The model under review builds one solid part; all positions refer to its coordinate system, in mm. A direction names the side the tool comes from. Round coordinates to 2 decimals unless told otherwise and drop trailing zeros. Order: outer loops, then holes, each group sorted by start corner. A loop starts at its lowest first (then second) coordinate and runs counter-clockwise, first axis right, second up. Notation, with made-up numbers: (65, -3.5) -> (69, -3.5) arc R36 ccw to (69, 35.5) -> close; hole circle Ø1 at (66.5, 68.25). An arc over 180 degrees is marked (long way). Use a Markdown table: item, result. Add a question column.
```python
from build123d import *

# Parameters (mm, degrees)
SKETCH1_R             = 24
SKETCH1_R_2           = 20
BOSS_EXTRUDE1_DEPTH   = 10
BOSS_EXTRUDE1_2_DEPTH = 10
BOSS_EXTRUDE1_3_DEPTH = 10
BOSS_EXTRUDE1_4_DEPTH = 10
BOSS_EXTRUDE2_DEPTH   = 3
SKETCH3_W             = 121.220550743
SKETCH3_H             = 101.763820318
CUT_EXTRUDE1_DEPTH    = 10
SKETCH4_R             = 4.5
BOSS_EXTRUDE4_DEPTH   = 5
FILLET1_R             = 10


with BuildPart() as part:
    # Sketch1 → Boss-Extrude1 (new body)
    with BuildSketch(Plane(origin=(0, 0, 0), x_dir=(1, 0, 0), z_dir=(0, 1, 0))):
        with Locations(Location((-28, -48.497422612, 0), (0, 0, 270))):
            Circle(SKETCH1_R)
        with Locations(Location((-28, -48.497422612, 0), (0, 0, 270))):
            Circle(SKETCH1_R_2, mode=Mode.SUBTRACT)
    extrude(amount=BOSS_EXTRUDE1_DEPTH)



with BuildPart() as body_2:
    # Sketch1 → Boss-Extrude1 2 (new body)
    with BuildSketch(Plane(origin=(0, 0, 0), x_dir=(1, 0, 0), z_dir=(0, 1, 0))):
        with Locations(Location((0, 0, 0), (0, 0, 270))):
            Circle(SKETCH1_R)
        with Locations(Location((0, 0, 0), (0, 0, 270))):
            Circle(SKETCH1_R_2, mode=Mode.SUBTRACT)
    extrude(amount=BOSS_EXTRUDE1_2_DEPTH)


with BuildPart() as body_3:
    # Sketch1 → Boss-Extrude1 3 (new body)
    with BuildSketch(Plane(origin=(0, 0, 0), x_dir=(1, 0, 0), z_dir=(0, 1, 0))):
        with Locations(Location((28, -48.497422612, 0), (0, 0, 270))):
            Circle(SKETCH1_R)
        with Locations(Location((28, -48.497422612, 0), (0, 0, 270))):
            Circle(SKETCH1_R_2, mode=Mode.SUBTRACT)
    extrude(amount=BOSS_EXTRUDE1_3_DEPTH)


with BuildPart() as body_4:
    # Sketch1 → Boss-Extrude1 4 (new body)
    with BuildSketch(Plane(origin=(0, 0, 0), x_dir=(1, 0, 0), z_dir=(0, 1, 0))):
        with BuildLine():
            ThreePointArc((4.672620947, -29.633876113), (2.019237886, -33.497422612), (0, -37.727092998))
            ThreePointArc((0, -37.727092998), (-2.019237886, -33.497422612), (-4.672620947, -29.633876113))
            ThreePointArc((-4.672620947, -29.633876113), (0, -30), (4.672620947, -29.633876113))
        make_face()
    extrude(amount=BOSS_EXTRUDE1_4_DEPTH)


with BuildPart() as part_1:
    add(part.part)

    add(body_2.part)  # Boss-Extrude2 merges body 2

    add(body_3.part)  # Boss-Extrude2 merges body 3

    add(body_4.part)  # Boss-Extrude2 merges body 4
    # Sketch2 → Boss-Extrude2 (add)
    with BuildSketch(Plane(origin=(0, 10, 0), x_dir=(1, 0, 0), z_dir=(0, 1, 0))):
        with BuildLine():
            Line((-20, -32.516950024), (-20, -56.505922275))
            Line((-20, -56.505922275), (20, -56.505922275))
            Line((20, -56.505922275), (20, -32.516950024))
            ThreePointArc((20, -32.516950024), (0, -12.516950024), (-20, -32.516950024))
        make_face()
    extrude(amount=BOSS_EXTRUDE2_DEPTH)

    # Sketch3 → Cut-Extrude1 (cut)
    with BuildSketch(Plane.XZ):
        with Locations((1.216045651, 23.416680071)):
            Rectangle(SKETCH3_W, SKETCH3_H)
        Polygon((0, 0), (28, 48.497422612), (-28, 48.497422612), align=None, mode=Mode.SUBTRACT)
    extrude(amount=-CUT_EXTRUDE1_DEPTH, mode=Mode.SUBTRACT)

    # Sketch4 → Boss-Extrude4 (add)
    with BuildSketch(Plane(origin=(0, 13, 0), x_dir=(1, 0, 0), z_dir=(0, 1, 0))):
        with Locations(Location((0, -32.516950024, 0), (0, 0, 270))):
            Circle(SKETCH4_R)
        with BuildLine():
            Line((-10, -18.516950024), (10, -18.516950024))
            ThreePointArc((10, -18.516950024), (11.4, -19.916950024), (10, -21.316950024))
            Line((10, -21.316950024), (-10, -21.316950024))
            ThreePointArc((-10, -21.316950024), (-11.4, -19.916950024), (-10, -18.516950024))
        make_face()
        with BuildLine():
            Line((-15, -49.516950024), (15, -49.516950024))
            ThreePointArc((15, -49.516950024), (16.4, -50.916950024), (15, -52.316950024))
            Line((15, -52.316950024), (-15, -52.316950024))
            ThreePointArc((-15, -52.316950024), (-16.4, -50.916950024), (-15, -49.516950024))
        make_face()
    extrude(amount=BOSS_EXTRUDE4_DEPTH)

    # Fillet1
    fillet1_edges = [part_1.edges().sort_by_distance(p)[0] for p in [
        (-20, 11.5, 56.505922275),
        (20, 11.5, 56.505922275),
    ]]
    fillet(fillet1_edges, radius=FILLET1_R)


solid = part_1.part
```
Q1. Mouldability with a two-part tool opening along X and no side actions: class faces 5 (the flat face through (0, 15, 49.517)), 6 (the flat face through (-11.014, 4.93, 19.077)), 7 (the cylindrical face through (7.3, 4.93, 36.35)) as pulls with the +X half, pulls with the -X half, needs draft (parallel to the pull), parting line crosses it, or undercut.
Q2. Add section B-B (y = 8.25). Write out the cut boundary in (x, z).
Q3. Add section D-D (z = 34). Write out the cut boundary in (x, y), then the cut area to 3 significant figures.
Q4. Add section A-A (y = 16.25). Write out the cut boundary in (x, z), then the cut area to 3 significant figures.
Q5. Wall thickness on line 1 (Z direction, x = 9, y = 13.5); line 2 (Z direction, x = 3, y = 16); line 3 (X direction, y = 12.25, z = 47): over which ranges is each line inside the solid? List them lowest first. Write a range as [from, to].
Q6. Add section C-C (z = 39.5). Write out the cut boundary in (x, y).
Q7. Insertion check: pin 1 (2.5 mm diameter, centred on x = -3, y = 16.5, fed in from +Z); pin 2 (1.5 mm diameter, centred on x = 4, y = 14.5, fed in from -Z); pin 3 (2 mm diameter, centred on x = 12, y = 4.5, fed in from -Z). Each pin has a flat end and moves straight along its axis. Give the tip position at first contact, or say it passes through.
Q8. Machinability: for faces 1 (the flat face through (16.986, 4.93, 29.421)), 2 (the cylindrical face through (-16.4, 15.5, 50.9)), 3 (the flat face through (6, 5, 48.497)), 4 (the cylindrical face through (-7.1, 4.9, 36.7)), which of the approach directions +Z, -Z, +X, -X, +Y, -Y give a long, thin tool a straight path to every point of the face, cutting with its end or side? Answer none if there is none.
Report:
| question | item | result |
|---|---|---|
| 1 | face 5 | needs draft |
| 1 | face 6 | pulls with the -X half |
| 1 | face 7 | undercut |
| 2 | outline | (-18, 31.18) -> (-16, 27.71) arc R24 ccw to (-4, 48.5) -> (-8, 48.5) arc R20 cw to start; (-12, 20.78) -> (-10, 17.32) arc R20 cw to (10, 17.32) -> (12, 20.78) arc R24 ccw to start; (-4.67, 29.63) arc R30 cw to (4.67, 29.63) arc R30 cw to (0, 37.73) arc R30 cw to start; (4, 48.5) arc R24 ccw to (16, 27.71) -> (18, 31.18) arc R20 cw to (8, 48.5) -> close |
| 3 | outline | (-20, 10) -> (-14.22, 10) -> (-14.22, 0) -> (-8.87, 0) -> (-8.87, 10) -> (-1.74, 10) -> (-1.74, 0) -> (1.74, 0) -> (1.74, 10) -> (8.87, 10) -> (8.87, 0) -> (14.22, 0) -> (14.22, 10) -> (20, 10) -> (20, 13) -> (4.25, 13) -> (4.25, 18) -> (-4.25, 18) -> (-4.25, 13) -> (-20, 13) -> close |
| 3 | area | 304 mm² |
| 4 | outline | (-15, 49.52) -> (15, 49.52) arc R1.4 ccw to (15, 52.32) -> (-15, 52.32) arc R1.4 ccw to start; (-10, 18.52) -> (10, 18.52) arc R1.4 ccw to (10, 21.32) -> (-10, 21.32) arc R1.4 ccw to start; circle Ø9 at (0, 32.52) |
| 4 | area | 216 mm² |
| 5 | line 1 | z = [18.52, 21.32], [49.52, 52.32] |
| 5 | line 2 | z = [18.52, 21.32], [29.16, 35.87], [49.52, 52.32] |
| 5 | line 3 | x = [-19.99, 19.99] |
| 6 | outline | (-20, 10) -> (-10.14, 10) -> (-10.14, 0) -> (-5.75, 0) -> (-5.75, 10) -> (5.75, 10) -> (5.75, 0) -> (10.14, 0) -> (10.14, 10) -> (20, 10) -> (20, 13) -> (-20, 13) -> close |
| 7 | pin 1 | stops at z = 52.32 |
| 7 | pin 2 | stops at z = 18.52 |
| 7 | pin 3 | stops at z = 19.05 |
| 8 | face 1 | -Z, +X, -Y |
| 8 | face 2 | -X, +Y |
| 8 | face 3 | +Z, +X, -X, -Y |
| 8 | face 4 | -Y |
